Can you work these out from the drawing? Everything is in mm from the part's minimum corner. A direction names the side the tool comes from. Round coordinates to 2 decimals unless told otherwise and drop trailing zeros. Write each loop counter-clockwise with the first axis right and the second up, starting at its lowest first coordinate (ties: lowest second). Pieces come first, ordered by that corner, then holes. Notation, with made-up numbers: (33, 33) -> (81, 33) arc R18 ccw to (81, 49) -> close; hole circle Ø6 at (18, 44). An arc over 180 degrees is marked (long way). One line per question, with ' | ' between items. Start each with the question number.
1. Imagine slicing it at C-C, the plane y = 29. List the corners of the cut face in (x, z) for me, and give its area (3 significant figures).
2. Thinking about a two-plate mould opening in X: for the marked faces 3, 4, 5 and 6, which applies, released by +X, released by -X, zero draft, split by the parting line, or undercut?
3. For pin 1 Ø1 at (x, y) = (33.5, 22) entering from -Z; pin 2 Ø1 at (x, z) = (25.5, 43) entering from +Y; pin 3 Ø1 at (x, z) = (31, 35.5) entering from +Y, each with a flat end and sliding along its axis, tell me the tip position at first contact or that it passes through.
4. For the marked faces 1 and 2, which set-ups out of +Z, -Z, +X, -X, +Y, -Y let a thin tool reach every point of the face, with its end or its side?
5. If I drill on line 1 along X through (y, z) = (6.5, 12.5); line 2 along Y through (x, z) = (19, 40.5), over which ranges is the centre line in solid material (lowest first)? Write a range as [from, to].
6. Imagine slicing it at A-A, the plane z = 23. List the corners of the cut face in (x, y) for me, and give its area (3 significant figures).
7. Imagine slicing it at D-D, the plane z = 33.5. List the corners of the cut face in (x, y) for me.
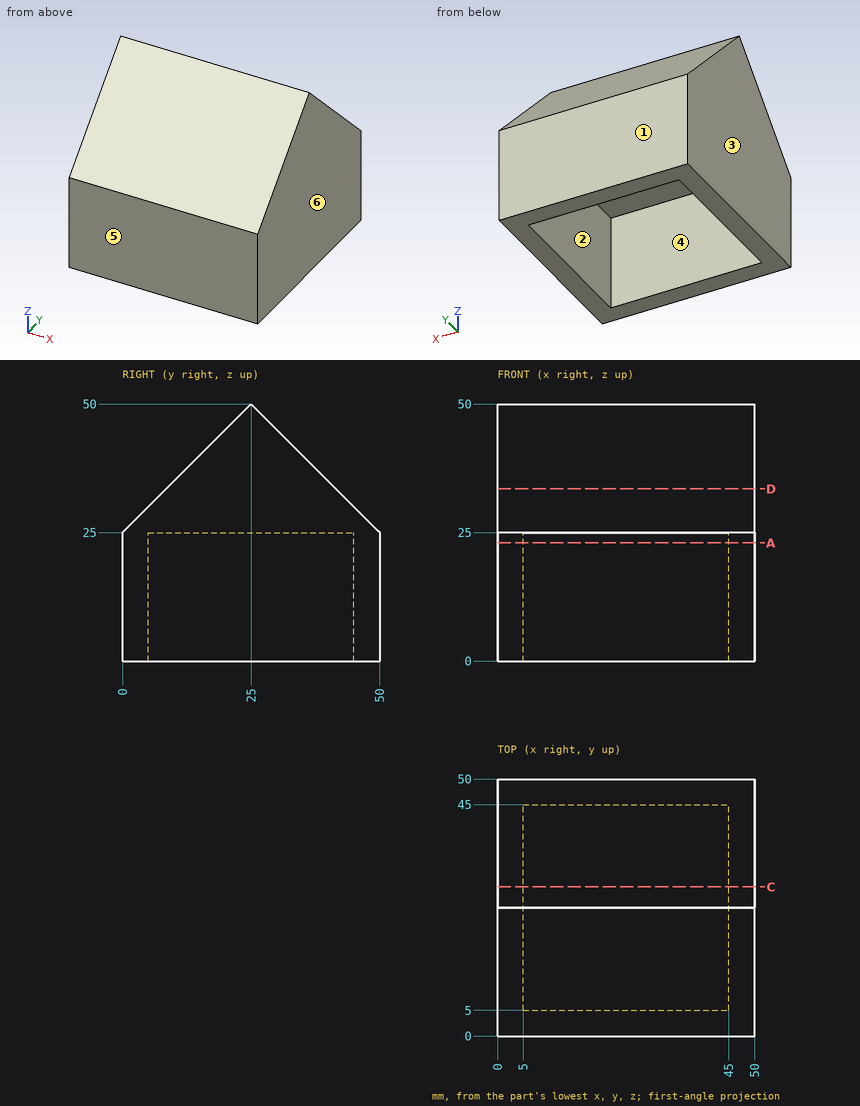
Geometry results:
1) outline: (0, 0) -> (5, 0) -> (5, 25) -> (45, 25) -> (45, 0) -> (50, 0) -> (50, 46) -> (0, 46) -> close | area: 1,300 mm2
2) face 3: released by -X | face 4: undercut | face 5: zero draft | face 6: released by +X
3) pin 1: stops at z = 25 | pin 2: stops at y = 32.5 | pin 3: stops at y = 40
4) face 1: +Z, -Z, +X, -X, +Y | face 2: -Z
5) line 1: x = [0, 5], [45, 50] | line 2: y = [15.5, 34.5]
6) outline: (0, 0) -> (50, 0) -> (50, 50) -> (0, 50) -> close; hole (5, 5) -> (45, 5) -> (45, 45) -> (5, 45) -> close | area: 900 mm2
7) outline: (0, 8.5) -> (50, 8.5) -> (50, 41.5) -> (0, 41.5) -> close
